Answer from the drawing. Dimensions are ordinates in mm from the lowest x, y and z of the part. Coordinates: 2 decimals unless noted, no trailing zeros. Write each loop counter-clockwise with the first axis right and the second up, starting at its lowest first coordinate (ties: lowest second). Pieces come first, ordered by that corner, then holes.
(1) Straight lines are drawn through the part: line 1 (Y direction, x = 68.5, z = 5.25); line 2 (X direction, y = 383, z = 4). For each, find the intervals that lie inside material, in ascending order.
(2) The part is cut by section A-A on x = 250. Determine the outline of the cut face in (y, z), plus the area to 3 significant figures.
(3) Given P1, Ø2, axis at y = 141, z = 4, coming from the -X side, flat-ended and moving along its own axis, determine where the tip first touches the part or whether it passes through.
(4) The part is cut by section C-C on z = 8. Determine the outline of the cut face in (x, y).
(5) The part is cut by section B-B on y = 176.5. Determine the outline of the cut face in (x, z), plus the area to 3 significant figures.
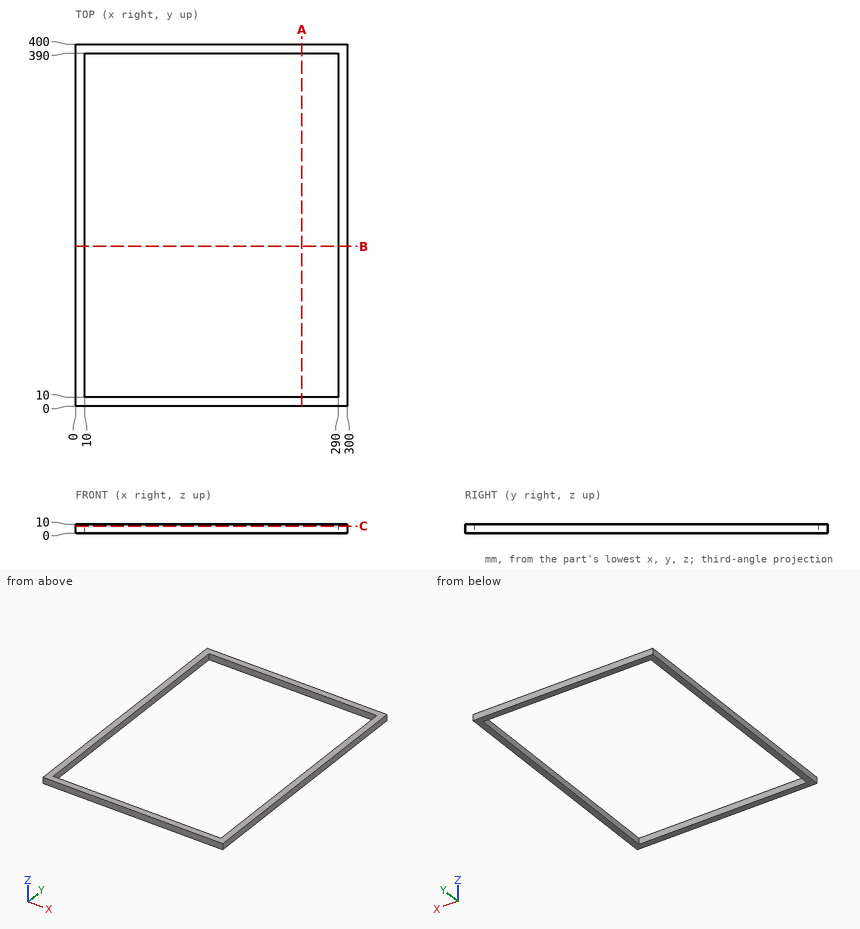
Model answer:
1. line 1: y = 0 to 10, 390 to 400
1. line 2: x = 0 to 10, 290 to 300
2. outline: (0, 0) - (10, 0) - (10, 10) - (0, 10) - close; (390, 0) - (400, 0) - (400, 10) - (390, 10) - close
2. area: 200 mm2
3. P1: stops at x = 0
4. outline: (0, 0) - (300, 0) - (300, 400) - (0, 400) - close; hole (10, 10) - (290, 10) - (290, 390) - (10, 390) - close
5. outline: (0, 0) - (10, 0) - (10, 10) - (0, 10) - close; (290, 0) - (300, 0) - (300, 10) - (290, 10) - close
5. area: 200 mm2
